```python
from build123d import *

# Parameters (mm, degrees)
BOSS_EXTRUDE1_DEPTH = 50.8
SKETCH2_W           = 12.7
SKETCH2_H           = 6.35
BOSS_EXTRUDE2_DEPTH = 6.35
SKETCH3_R           = 1.499997
CUT_EXTRUDE1_DEPTH  = 70.633186233
FILLET1_R           = 2.54
FILLET2_R           = 25.4
FILLET3_R           = 2.54


with BuildPart() as part:
    # Sketch1 → Boss-Extrude1 (new body)
    with BuildSketch(Plane(origin=(0, 0, 0), x_dir=(0, 0, -1), z_dir=(1, 0, 0))):
        Polygon((0, 0), (-41.275, 0), (-41.275, 3.175), (-3.175, 3.175), (-3.175, 28.575), (0, 28.575), align=None)
    extrude(amount=BOSS_EXTRUDE1_DEPTH)

    # Sketch2 → Boss-Extrude2 (add)
    with BuildSketch(Plane(origin=(0, 3.175, 0), x_dir=(1, 0, 0), z_dir=(0, 1, 0))):
        with Locations((25.4, -19.05)):
            Rectangle(SKETCH2_W, SKETCH2_H)
    extrude(amount=BOSS_EXTRUDE2_DEPTH)

    # Sketch3 → Cut-Extrude1 (cut, through all)
    with BuildSketch(Plane.XY.offset(3.175)):
        with Locations((25.4, 22.225)):
            Circle(SKETCH3_R)
    extrude(amount=-CUT_EXTRUDE1_DEPTH, mode=Mode.SUBTRACT)

    # Fillet1
    fillet1_edges = [part.edges().sort_by_distance(p)[0] for p in [
        (19.05, 9.525, 19.05),
        (25.4, 9.525, 22.225),
        (31.75, 9.525, 19.05),
        (25.4, 9.525, 15.875),
    ]]
    fillet(fillet1_edges, radius=FILLET1_R)

    # Fillet2
    fillet2_edges = [part.edges().sort_by_distance(p)[0] for p in [
        (0, 28.575, 1.5875),
        (50.8, 28.575, 1.5875),
        (50.8, 1.5875, 41.275),
        (0, 1.5875, 41.275),
    ]]
    fillet(fillet2_edges, radius=FILLET2_R - 0.0001)  # a hair under: the kernel refuses the full size

    # Fillet3
    fillet3_edges = [part.edges().sort_by_distance(p)[0] for p in [
        (25.4, 0, 0),
    ]]
    fillet(fillet3_edges, radius=FILLET3_R)


solid = part.part
```
CAD build for the part. Positions are in the model's coordinates, mm. A direction names the side the tool comes from. Round coordinates to 2 decimals unless told otherwise and drop trailing zeros. Order: outer loops, then holes, each group sorted by start corner. A loop starts at its lowest first (then second) coordinate and runs counter-clockwise, first axis right, second up. Notation, with made-up numbers: (17.5, -39.75) - (45.5, -39.75) arc R28 cw to (45.5, -0.75) - close; hole circle Ø4 at (-24, -29.5). An arc over 180 degrees is marked (long way). Answer as CSV lines item,"result". Start each with the question number.
1. Pull direction Z, two halves, no side cores. Call faces 4 (the face through (23.9, 22.3, 1.6)), 5 (the face through (25.49, 8.76, 16.6)), 6 (the face through (7.638, 1.61, 34.032)): +Z half, -Z half, draft (parallel to the pull), parting line (faces both ways), or undercut.
2. Tool access for faces 1 (the face through (19.05, 5, 19)), 2 (the face through (31.75, 5, 19)), 3 (the face through (25, 5, 22.225)): list every direction of +Z, -Z, +X, -X, +Y, -Y with a clear straight run to the whole face (end or side of a thin tool).
3. Saw through at C-C, the plane z = 17.5. Write the cut outline in (x, y) (3 decimals), and give its area (3 significant figures).
4. Saw through at D-D, the plane x = 4. Write the cut outline in (y, z) (3 decimals).
5. Pin check, flat tips, straight feed: pin 1 (12.5 mm diameter, centred on x = 18, y = 13, fed in from +Z) (3 decimals); pin 2 (1.8 mm diameter, centred on x = 25.4, y = 22.225, fed in from +Z); pin 3 (1.4 mm diameter, centred on x = 25, z = 19, fed in from +Y) (3 decimals); pin 4 (8 mm diameter, centred on x = 14, z = 25.5, fed in from +Y) (3 decimals). Stop position of each tip, or through.
6. Drill centre lines: L1, parallel to Z at x = 27, y = 4.75 (3 decimals); L2, parallel to Y at x = 25.4, z = 2.3 (3 decimals); L3, parallel to Y at x = 27, z = 10.5 (3 decimals). Where is each one in solid material? Low to high. Write a range as [from, to].
7. Saw through at A-A, the plane y = 4.25. Write the cut outline in (x, z) (3 decimals), and give its area (3 significant figures).
8. Saw through at B-B, the plane x = 41.5. Write the cut outline in (y, z) (3 decimals), and give its area (3 significant figures).
Model answer:
1,face 4,"draft"
1,face 5,"undercut"
1,face 6,"+Z half"
2,face 1,"+Z, -X, +Y"
2,face 2,"+Z, +X, +Y"
2,face 3,"+Z, +X, -X, +Y"
3,outline,"(0.052, 0) - (50.748, 0) - (50.748, 3.175) - (31.75, 3.175) - (31.75, 6.985) arc R2.54 ccw to (30.125, 9.354) - (20.675, 9.354) arc R2.54 ccw to (19.05, 6.985) - (19.05, 3.175) - (0.052, 3.175) - close"
3,area,"237 mm²"
4,outline,"(0, 2.54) arc R2.54 ccw to (2.54, 0) - (16.857, 0) - (16.857, 3.175) - (3.175, 3.175) - (3.175, 29.557) - (0, 29.557) - close"
5,pin 1,"stops at z = 22.225"
5,pin 2,"passes through"
5,pin 3,"stops at y = 9.525"
5,pin 4,"stops at y = 3.175"
6,L1,"z = [0, 3.175], [15.875, 22.225]"
6,L2,"y = [0.011, 20.725], [23.725, 28.575]"
6,L3,"y = [0, 3.175]"
7,outline,"(0.023, 0) - (50.777, 0) - (50.777, 3.175) - (0.023, 3.175) - close; (19.05, 15.875) - (31.75, 15.875) - (31.75, 22.225) - (19.05, 22.225) - close"
7,area,"242 mm²"
8,outline,"(0, 2.54) arc R2.54 ccw to (2.54, 0) - (22.821, 0) - (22.821, 3.175) - (3.175, 3.175) - (3.175, 35.521) - (0, 35.521) - close"
8,area,"174 mm²"
